Autodesk Inventor part; units mm, degrees
ref_plane "Work Plane1" through (-47.244, -26.7081, 1.651) normal (0, 0, 1) x (1, 0, 0)
ref_plane "YZ Plane" through (0, 0, 0) normal (1, 0, 0) x (0, 1, 0)
ref_plane "XZ Plane" through (0, 0, 0) normal (0, 1, 0) x (-1, 0, 0)
ref_plane "Work Plane1" through (-47.244, -26.7081, 1.651) normal (0, 0, 1) x (1, 0, 0)
sketch "Sketch1" plane through (-47.244, -26.7081, 1.651) normal (0, 0, 1) x (1, 0, 0)
  line L0 (-3.556, 38.1762) -> (-3.556, 3.556)
  line L1 (-1.016, 40.7162) -> (-3.556, 38.1762)
  line L2 (-3.556, 38.1762) -> (-1.016, 40.7162)
  line L3 (0.7474, 53.4162) -> (-1.016, 51.6528)
  line L4 (-1.016, 40.7162) -> (-1.016, 51.6528)
  line L5 (-1.016, 51.6528) -> (0.7474, 53.4162)
  line L6 (98.044, 51.8922) -> (96.52, 53.4162)
  line L7 (0.7474, 53.4162) -> (96.52, 53.4162)
  line L8 (96.52, 53.4162) -> (98.044, 51.8922)
  line L9 (96.52, 0) -> (98.044, 1.524)
  line L10 (98.044, 51.8922) -> (98.044, 1.524)
  line L11 (98.044, 1.524) -> (96.52, 0)
  line L12 (0, 0) -> (-3.556, 3.556)
  line L13 (96.52, 0) -> (0, 0)
  line L14 (0, 0) -> (-3.556, 3.556)
  line L15 (-3.556, 3.556) -> (-3.556, 38.1762)
  circle A0 centre (8.7884, 50.8762) radius 1.5621
  circle A1 centre (8.7884, 50.8762) radius 1.5
  circle A2 centre (83.9216, 50.8762) radius 1.5
  circle A3 centre (83.9216, 2.54) radius 1.5621
  circle A4 centre (83.9216, 2.54) radius 1.5
  circle A5 centre (1.2954, 2.54) radius 1.5621
  circle A6 centre (1.2954, 2.54) radius 1.5
  point P0 (47.244, 26.7081)
  dimension "d1" = 3
  dimension "d2" = 3
  dimension "d3" = 3
  dimension "d4" = 3
extrude "Extrusion1" add sketch "Sketch1" along normal blind 3 contours L1 L4 L3 L7 L6 L10 L9 L13 L12 L0
sketch "Sketch2" plane through (-47.244, -26.7081, 4.651) normal (0, 0, 1) x (1, 0, 0)
  line L0 (-3.556, 38.1762) -> (-3.556, 3.556)
  line L1 (-3.556, 3.556) -> (98.044, 3.556)
  line L2 (98.044, 3.556) -> (98.044, -11.444)
  line L3 (98.044, -11.444) -> (-3.556, -11.444)
  line L4 (-3.556, -11.444) -> (-3.556, 3.556)
  point P0 (47.244, 26.7081)
  dimension "d7" = 15
properties part number "arduino_holder"
Source: CAD feature listing. Evaluate the final solid. Frame: model axes, mm. A direction names the side the tool comes from. Coordinates: 2 decimals unless noted, no trailing zeros. Order: outer loops, then holes, each group sorted by start corner. A loop starts at its lowest first (then second) coordinate and runs counter-clockwise, first axis right, second up. Notation, with made-up numbers: M 48,-18 L 73,-18 A19 cw 73,12 Z; hole C 59.5,-10.5 d5. An arc over 180 degrees is marked long. Write each question's results on one line, items separated by ' | '. Start each with the question number.
Item 1: Line query: probe 1 along X at (y, z) = (15, 3.3). Output: solid intervals per line, ascending.
Item 2: First-contact query: pin 1 Ø1.9 at (x, y) = (-45.95, -24.17) entering from +Z; pin 2 Ø1.5 at (y, z) = (22, 3.5) entering from -X. Flat tips, straight axial feed; report the tip coordinate or a pass-through.
Item 3: Set-up query: faces 1 (the face through (-48.26, 19, 3)), 2 (the face through (50.8, 0, 3)). Return all of +Z, -Z, +X, -X, +Y, -Y with unobstructed straight access to the full face (end or side cutting, diameter ignored); none if empty.
Item 4: Draft query along Y for faces 3 (the face through (-47.366, 25.839, 3.13)), 4 (the face through (-50.8, -6, 3)), 5 (the face through (35.438, -23.218, 3.13)), 6 (the face through (35.18, 24.1, 3.13)). Return one class per face: pulls with the +Y half, pulls with the -Y half, needs draft (parallel to the pull), parting line crosses it, or undercut.
Item 5: Cut plane A-A (y = 19). Return loops of the section in (x, z).
Checked values:
1) probe 1: x = -48.26 to 50.8
2) pin 1: passes through | pin 2: stops at x = -48.26
3) face 1: +Z, -Z, -X, +Y | face 2: +Z, -Z, +X, +Y, -Y
4) face 3: pulls with the +Y half | face 4: needs draft | face 5: undercut | face 6: undercut
5) outline: M -48.26,1.65 L 50.8,1.65 L 50.8,4.65 L -48.26,4.65 Z
